Read the model definition and answer for the solid it produces. Units are mm, in the model's axes. A direction names the side the tool comes from. Coordinates: 2 decimals unless noted, no trailing zeros. Write each loop counter-clockwise with the first axis right and the second up, starting at its lowest first coordinate (ties: lowest second). Pieces come first, ordered by that corner, then holes. Notation, with made-up numbers: (10, -35.75) -> (66, -35.75) arc R9 cw to (66, -26.75) -> close; hole circle Ø10 at (-31.75, 64). An arc over 180 degrees is marked (long way). Return JSON: item names as keys, results as strings.
from build123d import *

# Parameters (mm, degrees)
F1_DEPTH       = 30
F3_W           = 27.5
F3_H           = 26
F4_DEPTH       = 37
F7_DEPTH       = 20.001
F9_W           = 13.75
F9_H           = 26
F10_W          = 13.75
F10_H          = 26
F11_DEPTH      = 5
F8_R           = 1.6
F12_DEPTH      = 2.001
F12_DEPTH_BACK = 28.001
F13_W          = 32.5
F13_H          = 20
F14_DEPTH      = 20
F15_DEPTH      = 20
F17_DEPTH      = 10.001
F18_R          = 10
F19_R          = 5
F20_R          = 1
F21_T1_DEPTH   = 33
F21_T4_ANGLE   = 180
F21_T6_ANGLE   = 180
F21_T8_ANGLE   = 180
F21_T10_ANGLE  = 180


# Not quite as in the source:
# - a fillet or chamfer that OpenCascade refuses, or shapes differently, is made with other operations: its cross-section is extruded or revolved along the edge and cut away or added


with BuildPart() as f1:
    # F0 (on Top) → F1 (new body)
    with BuildSketch(Plane.XY):
        with BuildLine():
            Line((-52.7744764373, 20.2577475536), (-52.7744764373, 0.2577475536))
            Line((-52.7744764373, 0.2577475536), (-22.7744764373, 0.2577475536))
            ThreePointArc((-22.7744764373, 0.2577475536), (19.7255235627, 32.8669618037), (62.2255235627, 0.2577475536))
            Line((62.2255235627, 0.2577475536), (92.2255235627, 0.2577475536))
            Line((92.2255235627, 0.2577475536), (92.2255235627, 20.2577475536))
            Line((92.2255235627, 20.2577475536), (72.2255235627, 20.2577475536))
            Line((72.2255235627, 20.2577475536), (72.2255235627, 40.2577475536))
            Line((72.2255235627, 40.2577475536), (52.2255235627, 40.2577475536))
            Line((52.2255235627, 40.2577475536), (52.2255235627, 65.2577475536))
            Line((52.2255235627, 65.2577475536), (-12.7744764373, 65.2577475536))
            Line((-12.7744764373, 65.2577475536), (-12.7744764373, 40.2577475536))
            Line((-12.7744764373, 40.2577475536), (-32.7744764373, 40.2577475536))
            Line((-32.7744764373, 40.2577475536), (-32.7744764373, 20.2577475536))
            Line((-32.7744764373, 20.2577475536), (-52.7744764373, 20.2577475536))
        make_face()
    extrude(amount=F1_DEPTH)

    # F3 (on offset) → F4 (cut)
    with BuildSketch(Plane.XZ.offset(-0.2577475536)):
        with Locations((-9.0244764373, 15)):
            Rectangle(F3_W, F3_H)
        with Locations((48.4755235627, 15)):
            Rectangle(F3_W, F3_H)
    extrude(amount=-F4_DEPTH, mode=Mode.SUBTRACT)

    # F6 (on face) + F5 (on face) → F7 (cut, through all)
    with BuildSketch(Plane(origin=(0, 20.2577475536, 0), x_dir=(-1, 0, 0), z_dir=(0, 1, 0))):
        Polygon((-86.3255235627, 17.3671361037), (-86.3255235627, 12.6328638963), (-82.2255235627, 10.2657277926), (-78.1255235627, 12.6328638963), (-78.1255235627, 17.3671361037), (-82.2255235627, 19.7342722074), align=None)
    with BuildSketch(Plane(origin=(0, 20.2577475536, 0), x_dir=(-1, 0, 0), z_dir=(0, 1, 0))):
        Polygon((42.7744764373, 10.2657277926), (46.8744764373, 12.6328638963), (46.8744764373, 17.3671361037), (42.7744764373, 19.7342722074), (38.6744764373, 17.3671361037), (38.6744764373, 12.6328638963), align=None)
    extrude(amount=-F7_DEPTH, mode=Mode.SUBTRACT)

    # F9 (on face) + F10 (on face) → F11 (cut)
    with BuildSketch(Plane.XZ.offset(-37.2577475536)):
        with Locations((41.6005235627, 15)):
            Rectangle(F9_W, F9_H)
    with BuildSketch(Plane.XZ.offset(-37.2577475536)):
        with Locations((-2.1494764373, 15)):
            Rectangle(F10_W, F10_H)
    extrude(amount=-F11_DEPTH, mode=Mode.SUBTRACT)

    # F8 (on face) → F12 (cut, two sides)
    with BuildSketch(Plane(origin=(0, 0, 28), x_dir=(1, 0, 0), z_dir=(0, 0, -1))) as f12_sk:
        with Locations((55.2255235627, -19.3357891615)):
            Circle(F8_R)
        with Locations((41.7255235627, -31.033055583)):
            Circle(F8_R)
        with Locations((-15.7744764373, -19.3357891615)):
            Circle(F8_R)
        with Locations((-2.2744764373, -31.033055583)):
            Circle(F8_R)
    extrude(amount=-F12_DEPTH, mode=Mode.SUBTRACT)
    extrude(f12_sk.sketch, amount=F12_DEPTH_BACK, mode=Mode.SUBTRACT)

    # F13 (on face) → F14 (cut)
    with BuildSketch(Plane(origin=(0, 0, 0), x_dir=(1, 0, 0), z_dir=(0, 0, -1))):
        with Locations((3.4755235627, -55.2577475536)):
            Rectangle(F13_W, F13_H)
    extrude(amount=-F14_DEPTH, mode=Mode.SUBTRACT)

    # F15 (add, through all): a face of the model
    f15_faces = [f1.faces().sort_by_distance(p)[0] for p in [
        (-12.7744764373, 49.9006046965, 20.7142857143),
    ]]
    extrude(f15_faces, amount=F15_DEPTH)

    # F16 (on face) → F17 (cut, through all)
    with BuildSketch(Plane(origin=(0, 0, 20), x_dir=(1, 0, 0), z_dir=(0, 0, -1))):
        with BuildLine():
            Line((-28.2744764373, -58.2577475536), (4.7255235627, -58.2577475536))
            ThreePointArc((4.7255235627, -58.2577475536), (7.7255235627, -55.2577475536), (4.7255235627, -52.2577475536))
            Line((4.7255235627, -52.2577475536), (-28.2744764373, -52.2577475536))
            ThreePointArc((-28.2744764373, -52.2577475536), (-31.2744764373, -55.2577475536), (-28.2744764373, -58.2577475536))
        make_face()
    extrude(amount=-F17_DEPTH, mode=Mode.SUBTRACT)

    # F18
    f18_edges = [f1.edges().sort_by_distance(p)[0] for p in [
        (52.225524, 65.257748, 15),
        (72.225524, 40.257748, 15),
    ]]
    fillet(f18_edges, radius=F18_R)

    # F19
    f19_edges = [f1.edges().sort_by_distance(p)[0] for p in [
        (52.225524, 40.257748, 15),
        (-32.774476, 65.257748, 25),
        (-32.774476, 45.257748, 10),
    ]]
    fillet(f19_edges, radius=F19_R)

    # F20
    f20_edges = [f1.edges().sort_by_distance(p)[0] for p in [
        (82.225524, 20.257748, 30),
        (92.225524, 10.257748, 30),
        (77.225524, 0.257748, 30),
        (92.225524, 0.257748, 15),
        (77.225524, 0.257748, 0),
        (92.225524, 10.257748, 0),
        (82.225524, 20.257748, 0),
        (92.225524, 20.257748, 15),
        (72.225524, 20.257748, 15),
        (-42.774476, 20.257748, 30),
        (-37.774476, 0.257748, 30),
        (-52.774476, 10.257748, 30),
        (-52.774476, 20.257748, 15),
        (-52.774476, 0.257748, 15),
        (-37.774476, 0.257748, 0),
        (-52.774476, 10.257748, 0),
        (-42.774476, 20.257748, 0),
        (-32.774476, 20.257748, 15),
        (19.725524, 55.257748, 0),
        (19.725524, 65.257748, 10),
        (-4.024476, 65.257748, 20),
        (59.725524, 40.257748, 0),
        (53.68999, 41.722214, 0),
        (69.296591, 37.328815, 0),
        (52.225524, 50.257748, 0),
        (72.225524, 25.257748, 0),
        (49.296591, 62.328815, 0),
        (30.975524, 65.257748, 0),
        (-4.024476, 45.257748, 0),
        (-31.31001, 43.793281, 0),
        (-32.774476, 30.257748, 0),
        (59.725524, 40.257748, 30),
        (53.68999, 41.722214, 30),
        (69.296591, 37.328815, 30),
        (52.225524, 50.257748, 30),
        (72.225524, 25.257748, 30),
        (49.296591, 62.328815, 30),
        (7.225524, 65.257748, 30),
        (-32.774476, 42.757748, 20),
        (-32.774476, 40.257748, 30),
        (-32.774476, 52.757748, 20),
        (-31.31001, 63.793281, 30),
        (-31.31001, 63.793281, 20),
    ]]
    fillet(f20_edges, radius=F20_R)

    # F21: chamfer of 1 on 8 edges, made by hand

    # F21_s2 → F21_t1 (cut)
    with BuildSketch(Plane.YZ.offset(-28.2744764373)):
        Polygon((58.2577475536, 21), (59.2577475536, 20), (58.2577475536, 20), align=None)
        Polygon((52.2577475536, 21), (51.2577475536, 20), (52.2577475536, 20), align=None)
        Polygon((59.2577475536, 30), (58.2577475536, 29), (58.2577475536, 30), align=None)
        Polygon((51.2577475536, 30), (52.2577475536, 29), (52.2577475536, 30), align=None)
    extrude(amount=F21_T1_DEPTH, mode=Mode.SUBTRACT)

    # F21_s3 → F21_t4 (revolve, cut)
    with BuildSketch(Plane.YZ.offset(4.7255235627)):
        Polygon((58.2577475536, 21), (59.2577475536, 20), (58.2577475536, 20), align=None)
    revolve(axis=Axis((4.7255235627, 55.2577475536, 20), (0, 0, -1)), revolution_arc=F21_T4_ANGLE, mode=Mode.SUBTRACT)

    # F21_s5 → F21_t6 (revolve, cut)
    with BuildSketch(Plane.YZ.offset(-28.2744764373)):
        Polygon((52.2577475536, 21), (51.2577475536, 20), (52.2577475536, 20), align=None)
    revolve(axis=Axis((-28.2744764373, 55.2577475536, 20), (0, 0, -1)), revolution_arc=F21_T6_ANGLE, mode=Mode.SUBTRACT)

    # F21_s7 → F21_t8 (revolve, cut)
    with BuildSketch(Plane.YZ.offset(-28.2744764373)):
        Polygon((51.2577475536, 30), (52.2577475536, 29), (52.2577475536, 30), align=None)
    revolve(axis=Axis((-28.2744764373, 55.2577475536, 30), (0, 0, -1)), revolution_arc=F21_T8_ANGLE, mode=Mode.SUBTRACT)

    # F21_s9 → F21_t10 (revolve, cut)
    with BuildSketch(Plane.YZ.offset(4.7255235627)):
        Polygon((59.2577475536, 30), (58.2577475536, 29), (58.2577475536, 30), align=None)
    revolve(axis=Axis((4.7255235627, 55.2577475536, 30), (0, 0, -1)), revolution_arc=F21_T10_ANGLE, mode=Mode.SUBTRACT)


solid = f1.part
1. The part is cut by section A-A (x = -26). Determine the outline of the cut face in (y, z), then the cut area to 3 significant figures.
Taken from the geometry:
{"outline": "(0.26, 1) arc R1 ccw to (1.26, 0) -> (44.26, 0) arc R1 ccw to (45.26, 1) -> (45.26, 20) -> (51.26, 20) -> (52.26, 21) -> (52.26, 29) -> (51.26, 30) -> (1.26, 30) arc R1 ccw to (0.26, 29) -> close; (58.26, 21) -> (59.26, 20) -> (64.26, 20) arc R1 ccw to (65.26, 21) -> (65.26, 29) arc R1 ccw to (64.26, 30) -> (59.26, 30) -> (58.26, 29) -> close", "area": "1,490 mm2"}
2. Flat-ended cylindrical pins translate along their axes: pin 1 Ø10 at (y, z) = (55.5, 15.5) entering from -X; pin 2 Ø4.5 at (y, z) = (26.5, 14.5) entering from +X; pin 3 Ø1 at (y, z) = (39, 17) entering from +X. Find the tip coordinate at first contact, or state that the pin passes through.
Taken from the geometry:
{"pin 1": "stops at x = -32.64", "pin 2": "stops at x = 72.23", "pin 3": "stops at x = 67.89"}
3. A tool of negligible diameter and unlimited length cuts with its end or side. For faces 3 (the face through (84.247, 10.398, 18.567)), 4 (the face through (-9.024, 40, 15)), 5 (the face through (-31.35, 43.75, 11.14)), 6 (the face through (60, 40.258, 15)), 7 (the face through (-12, 58.258, 25)), from which of +Z, -Z, +X, -X, +Y, -Y can it reach the whole face along a straight path? Write none if from no direction.
Taken from the geometry:
{"face 3": "+Y, -Y", "face 4": "-Y", "face 5": "-Z, -X, +Y", "face 6": "+Z, -Z, +X, +Y", "face 7": "+Z, -Z"}
4. For a pull along Z with two mould halves and no side action, classify faces 1 (the face through (-40.753, 10.398, 18.567)), 2 (the face through (69.218, 37.406, 15.196)) as +Z half, -Z half, draft (parallel to the pull), parting line (faces both ways), or undercut.
Taken from the geometry:
{"face 1": "undercut", "face 2": "draft"}
5. Consider L1, parallel to X at y = 24, z = 6; L2, parallel to X at y = 39, z = 27; L3, parallel to X at y = 7, z = 5.5. Determine where each line is inside the solid, lowest interval first.
Taken from the geometry:
{"L1": "x = -32.77 to -22.77, 62.23 to 72.23", "L2": "x = -32.77 to -9.02, 4.73 to 34.73, 48.48 to 67.08", "L3": "x = -52.77 to -22.77, 62.23 to 92.23"}
6. The part is cut by section C-C (y = 25). Determine the outline of the cut face in (x, z).
Taken from the geometry:
{"outline": "(-32.77, 1) arc R1 ccw to (-31.77, 0) -> (-5.38, 0) -> (-5.38, 2) -> (-22.77, 2) -> (-22.77, 28) -> (-5.38, 28) -> (-5.38, 30) -> (-31.77, 30) arc R1 ccw to (-32.77, 29) -> close; (44.83, 0) -> (71.23, 0) arc R1 ccw to (72.23, 1) -> (72.23, 29) arc R1 ccw to (71.23, 30) -> (44.83, 30) -> (44.83, 28) -> (62.23, 28) -> (62.23, 2) -> (44.83, 2) -> close"}
7. The part is cut by section B-B (y = 10). Count the separate pieces of the cut face and the enclosed holes in it, then the cut area to 3 significant figures.
Taken from the geometry:
{"separate pieces": "2", "enclosed holes": "2", "area": "1,710 mm2"}
